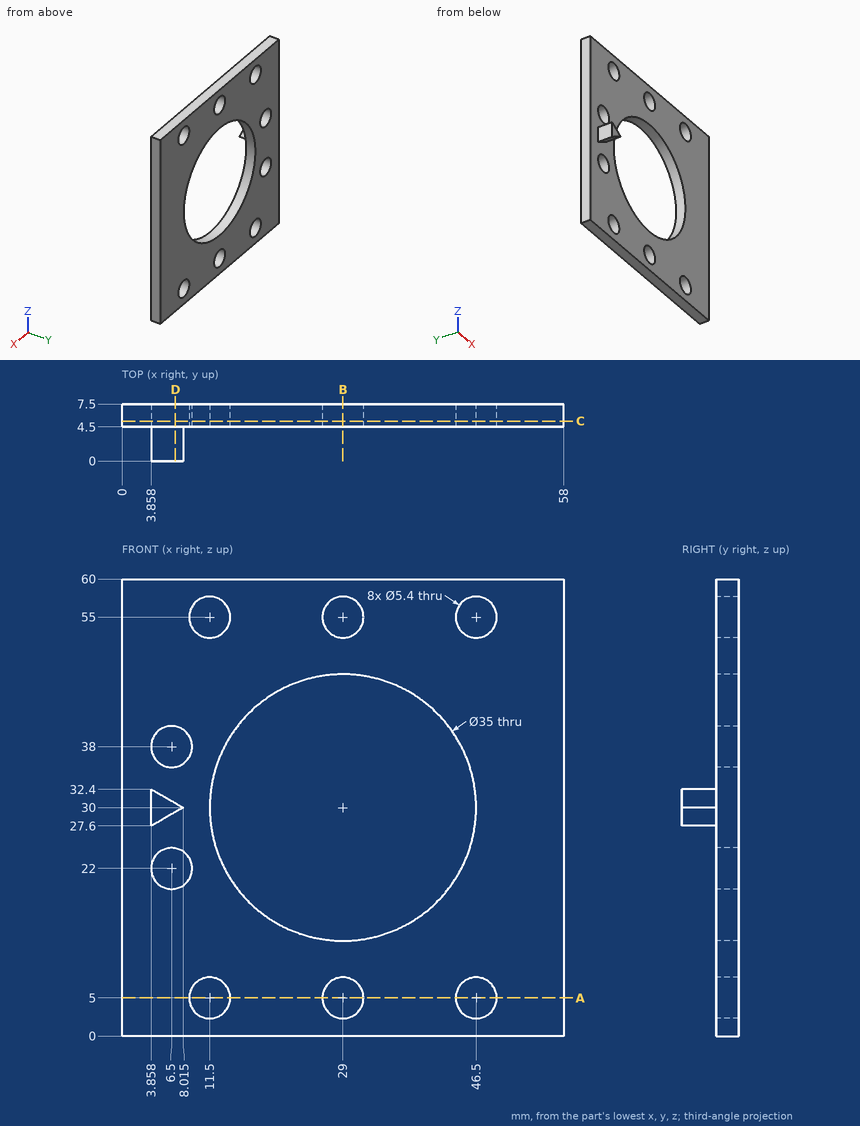
Drawing for the job (mm, zero at the part's lowest x, y, z). Round coordinates to 2 decimals unless told otherwise and drop trailing zeros. Order: outer loops, then holes, each group sorted by start corner. A loop starts at its lowest first (then second) coordinate and runs counter-clockwise, first axis right, second up.
Item 1: Saw through at D-D on x = 7. Write the cut outline in (y, z).
Item 2: Saw through at B-B on x = 29. Write the cut outline in (y, z), then the cut area to 3 significant figures.
Item 3: Saw through at A-A on z = 5. Write the cut outline in (x, y).
Item 4: Pin check, flat tips, straight feed: pin 1 (5 mm diameter, centred on x = 46.5, z = 55, fed in from +Y); pin 2 (1.5 mm diameter, centred on y = 3.5, z = 28, fed in from +X); pin 3 (6 mm diameter, centred on x = 11.5, z = 5, fed in from +Y); pin 4 (1.3 mm diameter, centred on y = 1.5, z = 30, fed in from -X). Stop position of each tip, or through.
Item 5: Probe line 1 along Z through (x, y) = (6.5, 6.1); line 2 along Z through (x, y) = (29, 5.3); line 3 along X through (y, z) = (7, 4.5). List the from-to ranges inside material, lowest first.
Item 6: Saw through at C-C on y = 5.25. State how many separate pieces and enclosed holes the cut face has, then the cut area to 3 significant figures.
Reported:
1. outline: (0, 29.41) - (4.5, 29.41) - (4.5, 24.65) - (7.5, 24.65) - (7.5, 35.35) - (4.5, 35.35) - (4.5, 30.59) - (0, 30.59) - close; (4.5, 0) - (7.5, 0) - (7.5, 19.35) - (4.5, 19.35) - close; (4.5, 40.65) - (7.5, 40.65) - (7.5, 60) - (4.5, 60) - close
2. outline: (4.5, 0) - (7.5, 0) - (7.5, 2.3) - (4.5, 2.3) - close; (4.5, 7.7) - (7.5, 7.7) - (7.5, 12.5) - (4.5, 12.5) - close; (4.5, 47.5) - (7.5, 47.5) - (7.5, 52.3) - (4.5, 52.3) - close; (4.5, 57.7) - (7.5, 57.7) - (7.5, 60) - (4.5, 60) - close
2. area: 42.6 mm2
3. outline: (0, 4.5) - (8.8, 4.5) - (8.8, 7.5) - (0, 7.5) - close; (14.2, 4.5) - (26.3, 4.5) - (26.3, 7.5) - (14.2, 7.5) - close; (31.7, 4.5) - (43.8, 4.5) - (43.8, 7.5) - (31.7, 7.5) - close; (49.2, 4.5) - (58, 4.5) - (58, 7.5) - (49.2, 7.5) - close
4. pin 1: passes through
4. pin 2: stops at x = 5.85
4. pin 3: stops at y = 7.5
4. pin 4: stops at x = 3.86
5. line 1: z = 0 to 19.3, 24.7 to 35.3, 40.7 to 60
5. line 2: z = 0 to 2.3, 7.7 to 12.5, 47.5 to 52.3, 57.7 to 60
5. line 3: x = 0 to 8.85, 14.15 to 26.35, 31.65 to 43.85, 49.15 to 58
6. separate pieces: 1
6. enclosed holes: 9
6. area: 2,330 mm2
